For this review, use the dimensioned drawing (mm, ordinates from the lowest corner) and the shaded views. A direction names the side the tool comes from. Round coordinates to 2 decimals unless told otherwise and drop trailing zeros. Loops run counter-clockwise (first coordinate to the right, second up) from the corner with the lowest first, then second, coordinate; pieces in that order, holes last. Notation, with made-up numbers: M 46,57.5 L 72,57.5 A25 ccw 72,91.5 Z; hole C 1.25,48.25 d7. An arc over 180 degrees is marked long. Write item = value, one per line. Start each with the question number.
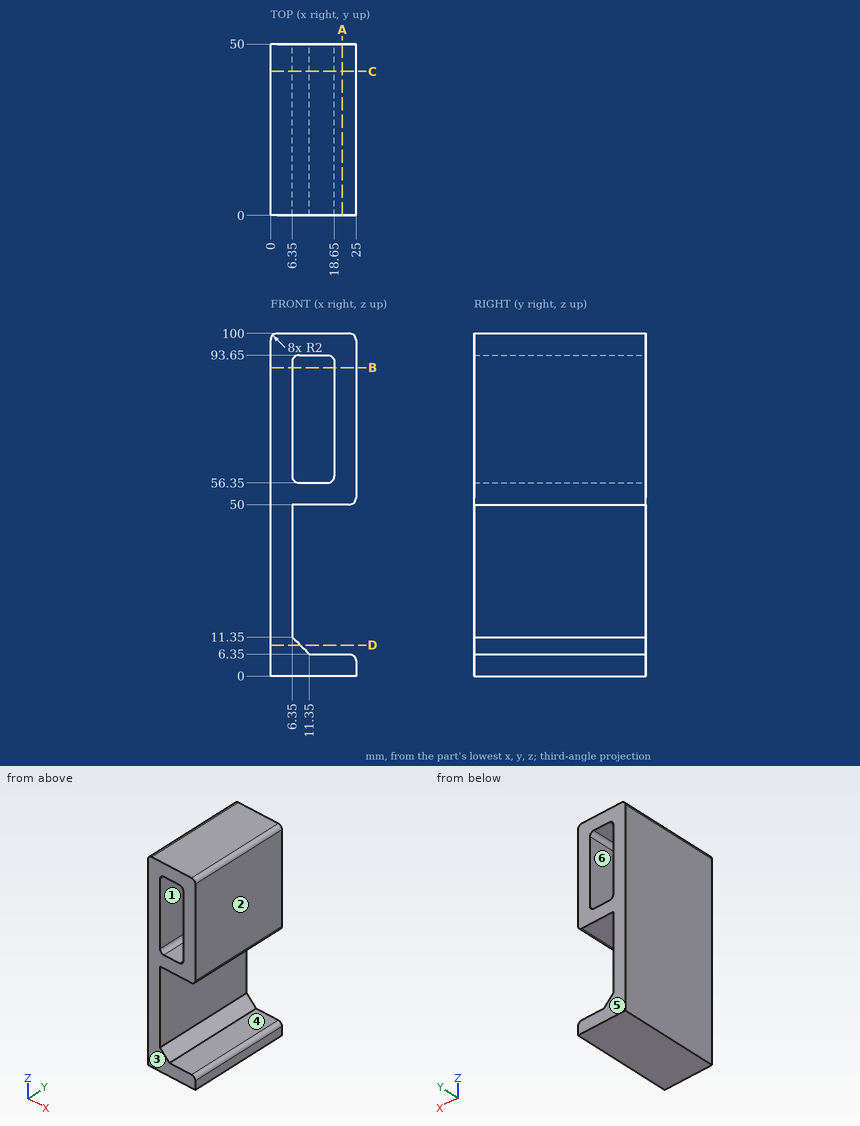
(1) Add section A-A on x = 21. Write out the cut boundary in (y, z).
(2) Wall thickness on L1, parallel to Z at x = 13.5, y = 2; L2, parallel to Z at x = 20, y = 24; L3, parallel to X at y = 13.5, z = 74: over which ranges is each line inside the solid? List them lowest first.
(3) Draft analysis for pull direction X (two halves, no side actions). For the marked faces 1, 2 and 3, state which applies: +X half, -X half, draft (parallel to the pull), parting line (faces both ways), or undercut.
(4) Tool access review of the marked faces 4, 5 and 6: name each direction out of +Z, -Z, +X, -X, +Y, -Y from which nothing blocks a thin tool from reaching the whole face with its end or side.
(5) Add section C-C on y = 42. Write out the cut boundary in (x, z), and give its area (3 significant figures).
(6) Add section B-B on z = 90. Write out the cut boundary in (x, y), and give its area (3 significant figures).
(7) Add section D-D on z = 9. Write out the cut boundary in (x, y).
Answer sheet:
q1.outline = M 0,0 L 50,0 L 50,6.35 L 0,6.35 Z; M 0,50 L 50,50 L 50,100 L 0,100 Z
q2.L1 = 0 to 6.35, 50 to 56.35, 93.65 to 100
q2.L2 = 0 to 6.35, 50 to 100
q2.L3 = 0 to 6.35, 18.65 to 25
q3.face_1 = undercut
q3.face_2 = +X half
q3.face_3 = draft
q4.face_4 = +X, +Y, -Y
q4.face_5 = +Z, -Z, +X, -X, +Y
q4.face_6 = +Y, -Y
q5.outline = M 0,0 L 25,0 L 25,4.35 A2 ccw 23,6.35 L 11.35,6.35 L 6.35,11.35 L 6.35,50 L 23,50 A2 ccw 25,52 L 25,98 A2 ccw 23,100 L 2,100 A2 ccw 0,98 Z; hole M 6.35,58.35 A2 ccw 8.35,56.35 L 16.65,56.35 A2 ccw 18.65,58.35 L 18.65,91.65 A2 ccw 16.65,93.65 L 8.35,93.65 A2 ccw 6.35,91.65 Z
q5.area = 1,240 mm²
q6.outline = M 0,0 L 6.35,0 L 6.35,50 L 0,50 Z; M 18.65,0 L 25,0 L 25,50 L 18.65,50 Z
q6.area = 635 mm²
q7.outline = M 0,0 L 8.7,0 L 8.7,50 L 0,50 Z
